Design review of the part built by this model. Coordinates are the model's own, in mm. Face numbers are marked on the shaded views. Coordinates: 2 decimals unless noted, no trailing zeros. Write each loop counter-clockwise with the first axis right and the second up, starting at its lowest first coordinate (ties: lowest second). Pieces come first, ordered by that corner, then holes. Notation, with made-up numbers: (-19, 82) -> (14, 82) arc R20 ccw to (14, 115) -> close; hole circle Ø5 at (-14.5, 70.5). An arc over 180 degrees is marked (long way). Answer in a Markdown table with one row per item. Add a question column.
Item 1: Clearance check with flat-ended pins moving along their axes: P1, Ø3.5, axis at x = 0, y = 31.5, coming from the +Z side; P2, Ø6.5, axis at x = 31, y = 0.5, coming from the +Z side; P3, Ø4.5, axis at x = -31.5, y = 0, coming from the +Z side; P4, Ø2, axis at x = 3, z = 2.5, coming from the +Y side. State where each tip first meets the part, or that it passes through.
Item 2: To check wall thickness, follow line 1 (Y direction, x = 0, z = 2.4); line 2 (X direction, y = 31.5, z = 3.15); line 3 (X direction, y = 16, z = 4.15). State the ranges of each line that lie inside material, in increasing order.
Item 3: Draft analysis for pull direction Y (two halves, no side actions). For the marked faces 1, 2 and 3, state which applies: released by +Y, released by -Y, zero draft, split by the parting line, or undercut.
Item 4: Take a section at D-D, the plane x = 31.5. Write out the cut boundary in (y, z).
Item 5: Take a section at C-C, the plane z = 3.3. Write out the cut boundary in (x, y), and give its area (3 significant figures).
Item 6: Take a section at B-B, the plane x = 0. Write out the cut boundary in (y, z).
Item 7: Take a section at A-A, the plane y = 0. Write out the cut boundary in (x, z), and give its area (3 significant figures).
Solid Edge part; units mm, degrees
sketch "Sketch1" plane through (0, 0, 0) normal (0, 0, 1) x (1, 0, 0)
  circle A0 centre (0, 0) radius 22.5
  circle A1 centre (0, 0) radius 35
extrude "Protrusion1" add sketch "Sketch1" along normal blind 5
hole "Hole_1" at (-31.5, 0, 5) direction (0, 0, -1) diameter 3.6 end up to next
hole "Hole1" at (0, 31.5, 5) direction (0, 0, -1) diameter 3.6 end up to next
hole "Hole2" at (31.5, 0, 5) direction (0, 0, -1) diameter 3.6 end up to next
hole "Hole_4" at (-31.5, 0, 5) direction (0, 0, -1) diameter 5.7 depth 3
hole "Hole3" at (0, 31.5, 5) direction (0, 0, -1) diameter 5.7 depth 3
hole "Hole4" at (31.5, 0, 5) direction (0, 0, -1) diameter 5.7 depth 3
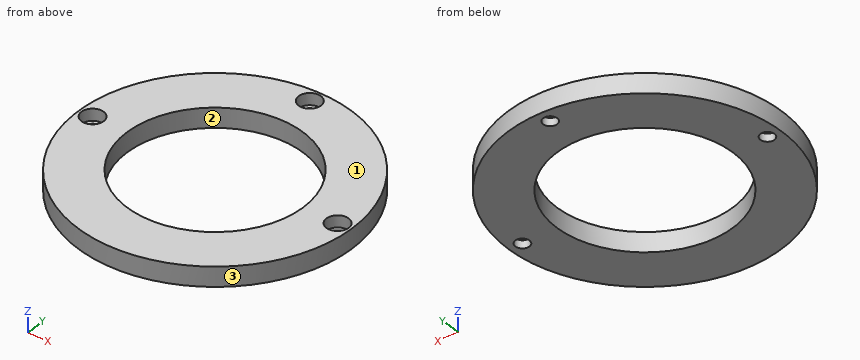
Answers:
| question | item | result |
|---|---|---|
| 1 | P1 | passes through |
| 1 | P2 | stops at z = 5 |
| 1 | P3 | stops at z = 2 |
| 1 | P4 | stops at y = 34.94 |
| 2 | line 1 | y = -35 to -22.5, 22.5 to 28.65, 34.35 to 35 |
| 2 | line 2 | x = -15.26 to -2.85, 2.85 to 15.26 |
| 2 | line 3 | x = -31.13 to -15.82, 15.82 to 31.13 |
| 3 | face 1 | zero draft |
| 3 | face 2 | undercut |
| 3 | face 3 | split by the parting line |
| 4 | outline | (-15.26, 0) -> (-1.8, 0) -> (-1.8, 2) -> (-2.85, 2) -> (-2.85, 5) -> (-15.26, 5) -> close; (1.8, 0) -> (15.26, 0) -> (15.26, 5) -> (2.85, 5) -> (2.85, 2) -> (1.8, 2) -> close |
| 5 | outline | circle Ø70 at (0, 0); hole circle Ø5.7 at (-31.5, 0); hole circle Ø45 at (0, 0); hole circle Ø5.7 at (0, 31.5); hole circle Ø5.7 at (31.5, 0) |
| 5 | area | 2,180 mm^2 |
| 6 | outline | (-35, 0) -> (-22.5, 0) -> (-22.5, 5) -> (-35, 5) -> close; (22.5, 0) -> (29.7, 0) -> (29.7, 2) -> (28.65, 2) -> (28.65, 5) -> (22.5, 5) -> close; (33.3, 0) -> (35, 0) -> (35, 5) -> (34.35, 5) -> (34.35, 2) -> (33.3, 2) -> close |
| 7 | outline | (-35, 0) -> (-33.3, 0) -> (-33.3, 2) -> (-34.35, 2) -> (-34.35, 5) -> (-35, 5) -> close; (-29.7, 0) -> (-22.5, 0) -> (-22.5, 5) -> (-28.65, 5) -> (-28.65, 2) -> (-29.7, 2) -> close; (22.5, 0) -> (29.7, 0) -> (29.7, 2) -> (28.65, 2) -> (28.65, 5) -> (22.5, 5) -> close; (33.3, 0) -> (35, 0) -> (35, 5) -> (34.35, 5) -> (34.35, 2) -> (33.3, 2) -> close |
| 7 | area | 76.4 mm^2 |
